Geometry: final body of the model. Coordinates: model frame, mm. A direction names the side the tool comes from. Round coordinates to 2 decimals unless told otherwise and drop trailing zeros. Loops run counter-clockwise (first coordinate to the right, second up) from the corner with the lowest first, then second, coordinate; pieces in that order, holes last. Notation, with made-up numbers: M 43,-32 L 83,-32 A12 cw 83,-11 Z; hole C -11.75,-31.75 d11. An arc over 180 degrees is marked long. Answer as a JSON object with one key per item and string values.
```python
from build123d import *

# Parameters (mm, degrees)
F0_W     = 63.144043088
F0_H     = 24.9639227986
F1_DEPTH = 25.4
F2_W     = 10.16
F2_H     = 1.27
F3_DEPTH = 3.175
F4_W     = 10.16
F4_H     = 1.27
F5_DEPTH = 3.175


# Not quite as in the source:
# - a feature names something its author has since deleted; it is built from what else it names


with BuildPart() as f1:
    # F0 (on Front) → F1 (new body, symmetric)
    with BuildSketch(Plane.XZ):
        Rectangle(F0_W, F0_H)
    extrude(amount=F1_DEPTH, both=True)

    # F2 (on Front) → F3 (join, symmetric)
    with BuildSketch(Plane.XZ):
        with Locations((36.6514939815, 9.6600476645)):
            Rectangle(F2_W, F2_H)
    extrude(amount=F3_DEPTH, both=True)

    # F4 (on Front) → F5 (join, symmetric)
    with BuildSketch(Plane.XZ):
        with Locations((-36.6476550698, -9.8343824477)):
            Rectangle(F4_W, F4_H)
    extrude(amount=F5_DEPTH, both=True)


solid = f1.part
```
1) Cut plane C-C on y = 19.5. Return the cut outline in (x, z).
Geometry results:
{"outline": "M -31.57,-12.48 L 31.57,-12.48 L 31.57,12.48 L -31.57,12.48 Z"}
2) Line query: probe 1 along X at (y, z) = (-9.5, 7); probe 2 along X at (y, z) = (3, -10); probe 3 along Z at (x, y) = (37, -2). Output: solid intervals per line, ascending.
Geometry results:
{"probe 1": "-31.57 to 31.57", "probe 2": "-41.73 to 31.57", "probe 3": "9.03 to 10.3"}
3) First-contact query: pin 1 (0.6 mm diameter, centred on x = -35.5, z = -10, fed in from +Y) (3 decimals); pin 2 (10 mm diameter, centred on y = 6, z = -1.5, fed in from -X); pin 3 (1.5 mm diameter, centred on y = 2.5, z = -8.5, fed in from +X). Flat tips, straight axial feed; report the tip coordinate or a pass-through.
Geometry results:
{"pin 1": "y = 3.175", "pin 2": "x = -31.57", "pin 3": "x = 31.57"}
4) Cut plane B-B on z = -1. Return the cut outline in (x, y), and give its area (3 significant figures).
Geometry results:
{"outline": "M -31.57,-25.4 L 31.57,-25.4 L 31.57,25.4 L -31.57,25.4 Z", "area": "3,210 mm2"}
5) Cut plane A-A on y = 0. Return the cut outline in (x, z), and give its area (3 significant figures).
Geometry results:
{"outline": "M -41.73,-10.47 L -31.57,-10.47 L -31.57,-12.48 L 31.57,-12.48 L 31.57,9.03 L 41.73,9.03 L 41.73,10.3 L 31.57,10.3 L 31.57,12.48 L -31.57,12.48 L -31.57,-9.2 L -41.73,-9.2 Z", "area": "1,600 mm2"}
6) Set-up query: faces 1 (the face through (37, 0, 9.025)), 2 (the face through (37, 0, 10.295)), 3 (the face through (-37, 0, -10.469)). Return all of +Z, -Z, +X, -X, +Y, -Y with unobstructed straight access to the full face (end or side cutting, diameter ignored); none if empty.
Geometry results:
{"face 1": "-Z, +X, +Y, -Y", "face 2": "+Z, +X, +Y, -Y", "face 3": "-Z, -X, +Y, -Y"}
